Here's how the part is built. I have some questions about the finished solid (model axes, mm). Face numbers are marked on the shaded views. A direction names the side the tool comes from. Round coordinates to 2 decimals unless told otherwise and drop trailing zeros. Order: outer loops, then holes, each group sorted by start corner. A loop starts at its lowest first (then second) coordinate and runs counter-clockwise, first axis right, second up.
```python
from build123d import *

# Parameters (mm, degrees)
PER_AGE1_D         = 6.6
BOSS_EXTRU_1_DEPTH = 70
ESQUISSE6_R        = 40
BOSS_EXTRU_2_DEPTH = 10
ESQUISSE7_R        = 40
BOSS_EXTRU_3_DEPTH = 20
BOSS_EXTRU_3_DRAFT = -30
ESQUISSE8_R        = 51.547005384
BOSS_EXTRU_4_DEPTH = 150
ESQUISSE9_R        = 51.547005384
BOSS_EXTRU_5_DEPTH = 20
BOSS_EXTRU_5_TAPER = 15
ESQUISSE10_R       = 20
BOSS_EXTRU_6_DEPTH = 5


with BuildPart() as part:
    # Esquisse1 → Base-Révolution (revolve)
    with BuildSketch(Plane.XY, mode=Mode.PRIVATE) as base_r_volution_sk:
        Polygon((30, 0), (35, 0), (35, -5), (52.5, -5), (52.5, -15), (35.8, -15), (25, -45), (0, -45), (0, -40), (21, -40), (30, -15), align=None)
    revolve(base_r_volution_sk.sketch.rotate(Axis((0, 32.384217016, 0), (0, -1, 0)), 90), axis=Axis((0, 32.384217016, 0), (0, -1, 0)))

    # Perçage1 (through all)
    with Locations(Plane(origin=(0, -5, 0), x_dir=(-1, 0, 0), z_dir=(0, 1, 0))):
        with Locations((42.5, 0), (-42.5, 0), (0, -42.5), (0, 42.5)):
            Hole(PER_AGE1_D / 2)

    # Esquisse2 → Boss.-Extru.1 (add)
    with BuildSketch(Plane.XZ.offset(45)):
        Polygon((-5, -40), (-5, -60), (-75, -60), (-75, 50), (-5, 50), (-5, 40), (40, 40), (40, -40), align=None)
    extrude(amount=BOSS_EXTRU_1_DEPTH)

    # Esquisse6 → Boss.-Extru.2 (add)
    with BuildSketch(Plane.XY.offset(50)):
        with Locations(Location((-40, -80, 0), (0, 0, 151.044975628))):
            Circle(ESQUISSE6_R)
    extrude(amount=BOSS_EXTRU_2_DEPTH)


with BuildPart() as boss_extru_3_tool:
    # Esquisse7 → Boss.-Extru.3 (with draft: the straight prism first)
    with BuildSketch(Plane.XY.offset(60)):
        with Locations(Location((-40, -80, 0), (0, 0, 151.044975628))):
            Circle(ESQUISSE7_R)
    extrude(amount=BOSS_EXTRU_3_DEPTH)
    # Boss.-Extru.3: the draft: its side faces are tilted about the plane it starts from
    boss_extru_3_sides = [boss_extru_3_tool.faces().sort_by_distance(p)[0] for p in [
        (-5, -99.364916731, 70),
    ]]
    draft(boss_extru_3_sides, Plane.XY.offset(60), BOSS_EXTRU_3_DRAFT)


with BuildPart() as part_1:
    add(part.part)

    # Boss.-Extru.3: add boss_extru_3_tool
    add(boss_extru_3_tool.part)

    # Esquisse8 → Boss.-Extru.4 (add)
    with BuildSketch(Plane.XY.offset(80)):
        with Locations((-40, -80)):
            Circle(ESQUISSE8_R)
    extrude(amount=BOSS_EXTRU_4_DEPTH)

    # Esquisse9 → Boss.-Extru.5 (add)
    with BuildSketch(Plane.XY.offset(230)):
        with Locations((-40, -80)):
            Circle(ESQUISSE9_R)
    extrude(amount=BOSS_EXTRU_5_DEPTH, taper=BOSS_EXTRU_5_TAPER)

    # Esquisse10 → Boss.-Extru.6 (add)
    with BuildSketch(Plane.XZ.offset(115)):
        with Locations(Location((0, 0, 0), (0, 0, 90))):
            Circle(ESQUISSE10_R)
    extrude(amount=BOSS_EXTRU_6_DEPTH)


solid = part_1.part
```
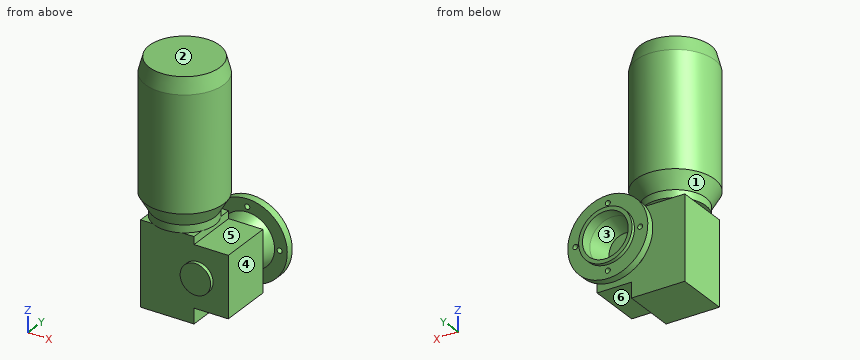
1) I need wall thicknesses on line 1 (Z direction, x = -1, y = -88); line 2 (X direction, y = -81, z = 15); line 3 (Y direction, x = -15.5, z = 28). Which ranges of each line are inside material? Lowest first, please.
2) We'd pull the mould along X, two halves only. Please class the marked faces 1, 2 and 3: +X half, -X half, draft (parallel to the pull), parting line (faces both ways), or undercut.
3) If we section it at A-A (z = 0): Give the number of separate pieces and of enclosed holes in the cut face, plus the area to 3 significant figures.
4) For the marked faces 4, 5 and 6, which set-ups out of +Z, -Z, +X, -X, +Y, -Y let a thin tool reach every point of the face, with its end or its side?
5) If we section it at B-B (z = 86): Write out the boundary of the cut face in (x, y), plus the area to 3 significant figures.
6) I'm going to push flat-ended pins straight in: pin 1 (4 mm diameter, centred on x = -69, z = 83, fed in from -Y); pin 2 (5.5 mm diameter, centred on x = -78.5, y = -77, fed in from -Z); pin 3 (8 mm diameter, centred on y = -97.5, z = 208, fed in from -X). Where does each tip first touch, or does it pass through?
Solutions:
1. line 1: z = -40 to 40, 50 to 250
1. line 2: x = -75 to 40
1. line 3: y = -115 to -45, -25.54 to 0
2. face 1: parting line
2. face 2: draft
2. face 3: undercut
3. separate pieces: 3
3. enclosed holes: 0
3. area: 9,170 mm2
4. face 4: +Z, -Z, +X, -Y
4. face 5: +X, -Y
4. face 6: -Z, +X, -Y
5. outline: circle Ø103.09 at (-40, -80)
5. area: 8,350 mm2
6. pin 1: stops at y = -123.91
6. pin 2: stops at z = 50
6. pin 3: stops at x = -89.75
